Work out the finished part from the listing and answer in its coordinate system (mm). Give positions to 0.01 mm unless a question says otherwise; leave off trailing zeros. Loops run counter-clockwise (first coordinate to the right, second up) from the corner with the lowest first, then second, coordinate; pieces in that order, holes last. Notation, with made-up numbers: M -23,-19 L -16,-19 A15 cw -16,3 Z; hole C -20.5,39 d3. An arc over 180 degrees is marked long. Answer in a Markdown table with one row per item. Add a question column.
from build123d import *

# Parameters (mm, degrees)
SKETCH_W         = 60
SKETCH_H         = 130
PAD_DEPTH        = 2.8
FILLET_R         = 1
FILLET001_R      = 1
FILLET002_R      = 1
FILLET003_R      = 1
SKETCH001_R      = 12
SKETCH001_R_2    = 1.7
POCKET_DEPTH     = 2.8
SKETCH002_W      = 40
SKETCH002_H      = 3
PAD001_DEPTH     = 52
SKETCH007_R      = 1.1
SKETCH007_W      = 24
SKETCH007_H      = 27.426216
POCKET003_DEPTH  = 3
SKETCH009_W      = 18
SKETCH009_H      = 8
PAD003_DEPTH     = 5
COPYSKETCH010_R  = 4
PAD004_DEPTH     = 6
SKETCH011_R      = 1.5
POCKET005_DEPTH  = 10
SKETCH013_R      = 1.7
POCKET006_DEPTH  = 2.8
SKETCH014_R      = 1.7
POCKET007_DEPTH  = 2.8
POCKET008_DEPTH  = 1
HOLE_D           = 3
HOLE_DEPTH       = 24.098709
HOLE_CSINK_D     = 7
HOLE_CSINK_ANGLE = 90
HOLE_TIPS_R      = 1.5


with BuildPart() as part:
    # Sketch → Pad (new body)
    with BuildSketch(Plane.XY):
        Rectangle(SKETCH_W, SKETCH_H)
    extrude(amount=PAD_DEPTH)

    # Fillet
    fillet_edges = [part.edges().sort_by_distance(p)[0] for p in [
        (-30, 65, 1.4),
    ]]
    fillet(fillet_edges, radius=FILLET_R)

    # Fillet001
    fillet001_edges = [part.edges().sort_by_distance(p)[0] for p in [
        (30, 65, 1.4),
    ]]
    fillet(fillet001_edges, radius=FILLET001_R)

    # Fillet002
    fillet002_edges = [part.edges().sort_by_distance(p)[0] for p in [
        (-30, -65, 1.4),
    ]]
    fillet(fillet002_edges, radius=FILLET002_R)

    # Fillet003
    fillet003_edges = [part.edges().sort_by_distance(p)[0] for p in [
        (30, -65, 1.4),
    ]]
    fillet(fillet003_edges, radius=FILLET003_R)

    # Sketch001 (on Face10 of Fillet003) → Pocket (cut)
    with BuildSketch(Plane.XY.offset(2.8)):
        with Locations((0, 40)):
            Circle(SKETCH001_R)
        with Locations((-22, 40)):
            Circle(SKETCH001_R_2)
        with Locations((22, 40)):
            Circle(SKETCH001_R_2)
        with Locations((-25, -35)):
            Circle(SKETCH001_R_2)
        with Locations((25, -35)):
            Circle(SKETCH001_R_2)
        with Locations((-25, 25)):
            Circle(SKETCH001_R_2)
        with Locations((25, 25)):
            Circle(SKETCH001_R_2)
    extrude(amount=-POCKET_DEPTH, mode=Mode.SUBTRACT)

    # Sketch002 (on Face1 of Pocket) → Pad001 (join)
    with BuildSketch(Plane(origin=(0, 0, 0), x_dir=(1, 0, 0), z_dir=(0, 0, -1))):
        with Locations((0, 53.5)):
            Rectangle(SKETCH002_W, SKETCH002_H)
    extrude(amount=PAD001_DEPTH)

    # Sketch007 (on Face20 of Pad001) → Pocket003 (cut)
    with BuildSketch(Plane(origin=(0, -52, 0), x_dir=(-1, 0, 0), z_dir=(0, 1, 0))):
        with Locations((-14, -48)):
            Circle(SKETCH007_R)
        with Locations((14, -48)):
            Circle(SKETCH007_R)
        with Locations((14, -20)):
            Circle(SKETCH007_R)
        with Locations((-14, -20)):
            Circle(SKETCH007_R)
        with Locations((0, -38.713108)):
            Rectangle(SKETCH007_W, SKETCH007_H)
    extrude(amount=-POCKET003_DEPTH, mode=Mode.SUBTRACT)

    # Sketch009 → Pad003 (join)
    with BuildSketch(Plane(origin=(0, -52, 0), x_dir=(-1, 0, 0), z_dir=(0, 1, 0))):
        with Locations((0, -4)):
            Rectangle(SKETCH009_W, SKETCH009_H)
    extrude(amount=PAD003_DEPTH)

    # CopySketch010 → Pad004 (join)
    with BuildSketch(Plane(origin=(0, 0, 0), x_dir=(1, 0, 0), z_dir=(0, 0, -1))):
        with Locations((0, 60.064695)):
            Circle(COPYSKETCH010_R)
    extrude(amount=PAD004_DEPTH)

    # Sketch011 (on Face26 of Pad004) → Pocket005 (cut)
    with BuildSketch(Plane(origin=(0, 0, -6), x_dir=(1, 0, 0), z_dir=(0, 0, -1))):
        with Locations((0, 60.064695)):
            Circle(SKETCH011_R)
    extrude(amount=-POCKET005_DEPTH, mode=Mode.SUBTRACT)

    # Sketch013 (on Face1 of Pocket005) → Pocket006 (cut)
    with BuildSketch(Plane(origin=(0, 0, 0), x_dir=(1, 0, 0), z_dir=(0, 0, -1))):
        with Locations((-4.986458, 44.510635)):
            Circle(SKETCH013_R)
        with Locations((4.992854, 44.491314)):
            Circle(SKETCH013_R)
        with Locations((-4.984121, 29.546223)):
            Circle(SKETCH013_R)
        with Locations((4.992854, 29.527281)):
            Circle(SKETCH013_R)
    extrude(amount=-POCKET006_DEPTH, mode=Mode.SUBTRACT)

    # Sketch014 (on Face29 of Pocket006) → Pocket007 (cut)
    with BuildSketch(Plane.XY.offset(2.8)):
        with Locations((0, 40)):
            Circle(SKETCH014_R)
        with Locations((-4.984121, -29.546223)):
            Circle(SKETCH014_R)
        with Locations((4.992854, -44.491314)):
            Circle(SKETCH014_R)
        with Locations((-4.986458, -44.510635)):
            Circle(SKETCH014_R)
        with Locations((4.992854, -29.527281)):
            Circle(SKETCH014_R)
    extrude(amount=-POCKET007_DEPTH, mode=Mode.SUBTRACT)

    # Sketch014 (on Face29 of Pocket006) → Pocket008 (cut)
    with BuildSketch(Plane.XY.offset(2.8)):
        with Locations((0, 40)):
            Circle(SKETCH014_R)
        with Locations((-4.984121, -29.546223)):
            Circle(SKETCH014_R)
        with Locations((4.992854, -44.491314)):
            Circle(SKETCH014_R)
        with Locations((-4.986458, -44.510635)):
            Circle(SKETCH014_R)
        with Locations((4.992854, -29.527281)):
            Circle(SKETCH014_R)
    extrude(amount=-POCKET008_DEPTH, mode=Mode.SUBTRACT)

    # Hole
    with Locations(Plane.XY.offset(2.8)):
        with Locations((0, 40), (-4.984121, -29.546223), (4.992854, -44.491314), (-4.986458, -44.510635), (4.992854, -29.527281)):
            CounterSinkHole(HOLE_D / 2, HOLE_CSINK_D / 2, depth=HOLE_DEPTH, counter_sink_angle=HOLE_CSINK_ANGLE)

    # Hole tips → Hole tip 1 section 0
    with BuildSketch(Plane.XY.offset(-21.298709), mode=Mode.PRIVATE) as hole_tip_1_s0:
        with Locations((0, 40)):
            Circle(HOLE_TIPS_R)
    loft([hole_tip_1_s0.sketch, Vertex(0, 40, -22.2)], mode=Mode.SUBTRACT)

    # Hole tips → Hole tip 2 section 0
    with BuildSketch(Plane.XY.offset(-21.298709), mode=Mode.PRIVATE) as hole_tip_2_s0:
        with Locations((-4.984121, -29.546223)):
            Circle(HOLE_TIPS_R)
    loft([hole_tip_2_s0.sketch, Vertex(-4.984121, -29.546223, -22.2)], mode=Mode.SUBTRACT)

    # Hole tips → Hole tip 3 section 0
    with BuildSketch(Plane.XY.offset(-21.298709), mode=Mode.PRIVATE) as hole_tip_3_s0:
        with Locations((4.992854, -44.491314)):
            Circle(HOLE_TIPS_R)
    loft([hole_tip_3_s0.sketch, Vertex(4.992854, -44.491314, -22.2)], mode=Mode.SUBTRACT)

    # Hole tips → Hole tip 4 section 0
    with BuildSketch(Plane.XY.offset(-21.298709), mode=Mode.PRIVATE) as hole_tip_4_s0:
        with Locations((-4.986458, -44.510635)):
            Circle(HOLE_TIPS_R)
    loft([hole_tip_4_s0.sketch, Vertex(-4.986458, -44.510635, -22.2)], mode=Mode.SUBTRACT)

    # Hole tips → Hole tip 5 section 0
    with BuildSketch(Plane.XY.offset(-21.298709), mode=Mode.PRIVATE) as hole_tip_5_s0:
        with Locations((4.992854, -29.527281)):
            Circle(HOLE_TIPS_R)
    loft([hole_tip_5_s0.sketch, Vertex(4.992854, -29.527281, -22.2)], mode=Mode.SUBTRACT)


solid = part.part
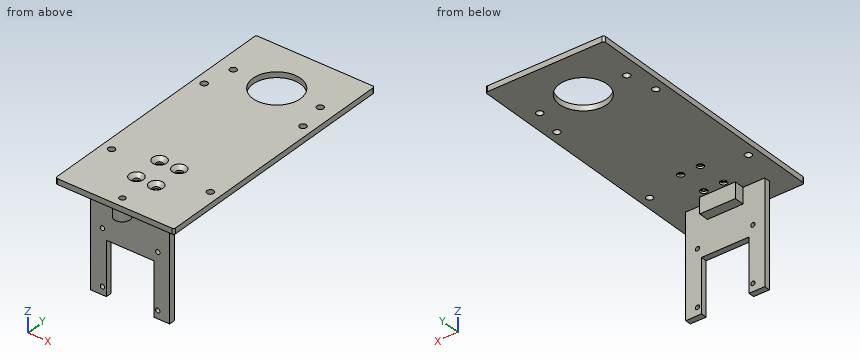
(1) Section A-A, the plane y = 40 is taken. Determine the outline of the cut face in (x, z).
(2) Section D-D, the plane z = -17 is taken. Determine the outline of the cut face in (x, y).
(3) Section C-C, the plane y = -35 is taken. Determine the outline of the cut face in (x, z).
(4) Consider line 1 along Y through (x, z) = (-25, 2.2); line 2 along Y through (x, z) = (19.5, -43); line 3 along Z through (x, y) = (1, 22). Determine where each line is inside the solid, lowest interval first. Write a range as from..to.
(5) Section B-B, the plane z = -39.5 is taken. Determine the outline of the cut face in (x, y).
(6) Each of these flat-tipped pins is pushed along its axis until it touches: P1, Ø1.5, axis at y = -50, z = -2, coming from the -X side; P2, Ø12, axis at x = 4, y = 38.5, coming from the -Z side; P3, Ø3, axis at x = -14, z = -20, coming from the -Y side; P4, Ø3.5, axis at y = -53.5, z = -35, coming from the -X side. Where does it stop, or does it pass through?
Numbers:
| question | item | result |
|---|---|---|
| 1 | outline | M -30,0 L -23.7,0 L -23.7,2.8 L -30,2.8 Z; M -20.3,0 L -12,0 L -12,2.8 L -20.3,2.8 Z; M 12,0 L 20.3,0 L 20.3,2.8 L 12,2.8 Z; M 23.7,0 L 30,0 L 30,2.8 L 23.7,2.8 Z |
| 2 | outline | M -20,-55 L 20,-55 L 20,-52 L -20,-52 Z |
| 3 | outline | M -30,0 L -26.7,0 L -26.7,2.8 L -30,2.8 Z; M -23.3,0 L 23.3,0 L 23.3,2.8 L -23.3,2.8 Z; M 26.7,0 L 30,0 L 30,2.8 L 26.7,2.8 Z |
| 4 | line 1 | y = -65..-36.7, -33.3..23.3, 26.7..65 |
| 4 | line 2 | y = -55..-52 |
| 4 | line 3 | z = 0..2.8 |
| 5 | outline | M -20,-55 L -12,-55 L -12,-52 L -20,-52 Z; M 12,-55 L 20,-55 L 20,-52 L 12,-52 Z |
| 6 | P1 | stops at x = -9 |
| 6 | P2 | passes through |
| 6 | P3 | stops at y = -55 |
| 6 | P4 | stops at x = -20 |
